from build123d import *

# Parameters (mm, degrees)
F0_W     = 7.8232
F0_H     = 6.35
F0_W_2   = 69.85
F0_H_2   = 3.175
F0_W_3   = 55.9308
F0_H_3   = 69.85
F0_W_4   = 7.7978
F0_H_4   = 12.7
F0_W_5   = 85.725
F1_DEPTH = 25.4
F0_W_6   = 2.8702
F0_H_5   = 5.1918955931
F0_W_7   = 66.0908
F0_H_6   = 4.9097025247
F0_H_7   = 13.4315382606
F0_W_8   = 16.764
F0_H_8   = 0.762
F2_DEPTH = 6.35


with BuildPart() as f1:
    # F0 (on Front) → F1 (new body)
    with BuildSketch(Plane.XZ):
        with Locations((148.4884, 43.5362195122)):
            Rectangle(F0_W, F0_H)
        with Locations((109.6518, 43.5362195122)):
            Rectangle(F0_W_2, F0_H)
        with Locations((148.4884, 38.7737195122)):
            Rectangle(F0_W, F0_H_2)
        with Locations((46.7614, 43.5362195122)):
            Rectangle(F0_W_3, F0_H)
        with Locations((109.6518, 38.7737195122)):
            Rectangle(F0_W_2, F0_H_2)
        with Locations((148.4884, 2.2612195122)):
            Rectangle(F0_W, F0_H_3)
        with Locations((46.7614, 38.7737195122)):
            Rectangle(F0_W_3, F0_H_2)
        with Locations((148.4884, -34.2512804878)):
            Rectangle(F0_W, F0_H_2)
        with Locations((-70.8279, 43.5362195122)):
            Rectangle(F0_W_4, F0_H)
        Polygon((74.7268, -2.1837804878), (74.7268, 37.1862195122), (18.796, 37.1862195122), (18.796, 3.0081151053), (18.796, -2.1837804878), align=None)
        with Locations((109.6518, -34.2512804878)):
            Rectangle(F0_W_2, F0_H_2)
        with Locations((148.4884, -39.0137804878)):
            Rectangle(F0_W, F0_H)
        with Locations((-109.6518, 43.5362195122)):
            Rectangle(F0_W_2, F0_H)
        with Locations((-70.8279, 38.7737195122)):
            Rectangle(F0_W_4, F0_H_2)
        with Locations((46.7614, -8.5337804878)):
            Rectangle(F0_W_3, F0_H_4)
        with Locations((109.6518, -39.0137804878)):
            Rectangle(F0_W_2, F0_H)
        Polygon((18.796, -32.6637804878), (74.7268, -32.6637804878), (74.7268, -14.8837804878), (18.796, -14.8837804878), (18.796, -28.3153187484), align=None)
        with Locations((46.7614, -34.2512804878)):
            Rectangle(F0_W_3, F0_H_2)
        with Locations((-148.4884, 43.5362195122)):
            Rectangle(F0_W, F0_H)
        with Locations((-109.6518, 38.7737195122)):
            Rectangle(F0_W_2, F0_H_2)
        Polygon((-66.929, 2.7259220369), (-66.929, 37.1862195122), (-74.7268, 37.1862195122), (-74.7268, -2.1837804878), (-66.929, -2.1837804878), align=None)
        with Locations((46.7614, -39.0137804878)):
            Rectangle(F0_W_3, F0_H)
        with Locations((-148.4884, 38.7737195122)):
            Rectangle(F0_W, F0_H_2)
        with Locations((-24.0665, -39.0137804878)):
            Rectangle(F0_W_5, F0_H)
        Polygon((-74.7268, -32.6637804878), (-66.929, -32.6637804878), (-66.929, -28.3153187484), (-66.929, -14.8837804878), (-74.7268, -14.8837804878), align=None)
        with Locations((-70.8279, -34.2512804878)):
            Rectangle(F0_W_4, F0_H_2)
        with Locations((-148.4884, 2.2612195122)):
            Rectangle(F0_W, F0_H_3)
        with Locations((-70.8279, -8.5337804878)):
            Rectangle(F0_W_4, F0_H_4)
        with Locations((-70.8279, -39.0137804878)):
            Rectangle(F0_W_4, F0_H)
        with Locations((-109.6518, -34.2512804878)):
            Rectangle(F0_W_2, F0_H_2)
        with Locations((-148.4884, -34.2512804878)):
            Rectangle(F0_W, F0_H_2)
        with Locations((-109.6518, -39.0137804878)):
            Rectangle(F0_W_2, F0_H)
        with Locations((-148.4884, -39.0137804878)):
            Rectangle(F0_W, F0_H)
    extrude(amount=F1_DEPTH)

    # F0 (on Front) → F2 (join)
    with BuildSketch(Plane.XZ):
        with Locations((-24.0665, 43.5362195122)):
            Rectangle(F0_W_5, F0_H)
        with Locations((-70.8279, 43.5362195122)):
            Rectangle(F0_W_4, F0_H)
        with Locations((-24.0665, 38.7737195122)):
            Rectangle(F0_W_5, F0_H_2)
        with Locations((-70.8279, 38.7737195122)):
            Rectangle(F0_W_4, F0_H_2)
        Polygon((18.796, 3.0081151053), (18.796, 37.1862195122), (-66.929, 37.1862195122), (-66.929, 2.7259220369), (-0.8382, 2.7259220369), (-0.8382, 3.0081151053), (15.9258, 3.0081151053), align=None)
        with Locations((17.3609, 0.4121673088)):
            Rectangle(F0_W_6, F0_H_5)
        Polygon((18.796, -14.8837804878), (18.796, -2.1837804878), (15.9258, -2.1837804878), (15.9258, -2.9457804878), (15.9258, -14.8837804878), align=None)
        Polygon((-66.929, -32.6637804878), (18.796, -32.6637804878), (18.796, -28.3153187484), (15.9258, -28.3153187484), (-0.8382, -28.3153187484), (-66.929, -28.3153187484), align=None)
        with Locations((-24.0665, -34.2512804878)):
            Rectangle(F0_W_5, F0_H_2)
        with Locations((-33.8836, 0.2710707746)):
            Rectangle(F0_W_7, F0_H_6)
        Polygon((15.9258, -2.1837804878), (15.9258, 3.0081151053), (-0.8382, 3.0081151053), (-0.8382, 2.7259220369), (-0.8382, -2.1837804878), align=None)
        with Locations((17.3609, -21.5995496181)):
            Rectangle(F0_W_6, F0_H_7)
        with Locations((7.5438, -2.5647804878)):
            Rectangle(F0_W_8, F0_H_8)
        Polygon((-0.8382, -2.1837804878), (-66.929, -2.1837804878), (-66.929, -14.8837804878), (-0.8382, -14.8837804878), (-0.8382, -2.9457804878), align=None)
        with Locations((7.5438, -21.5995496181)):
            Rectangle(F0_W_8, F0_H_7)
        with Locations((-33.8836, -21.5995496181)):
            Rectangle(F0_W_7, F0_H_7)
    extrude(amount=F2_DEPTH)


solid = f1.part
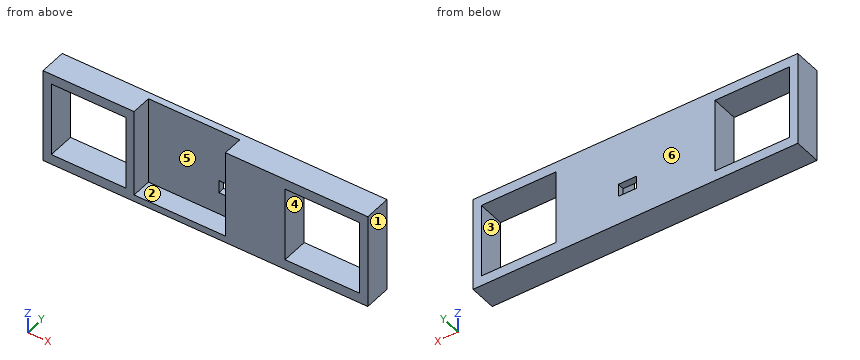
The model under review builds one solid part; all positions refer to its coordinate system, in mm. Face numbers are marked on the shaded views. A direction names the side the tool comes from. Round coordinates to 2 decimals unless told otherwise and drop trailing zeros. Write each loop counter-clockwise with the first axis right and the second up, starting at its lowest first coordinate (ties: lowest second). Pieces come first, ordered by that corner, then holes. Notation, with made-up numbers: M 54,55 L 113,55 A27 ccw 113,77 Z; hole C 54.25,-9 d1. An arc over 180 degrees is marked long. Answer as CSV lines item,"result". Start each with the question number.
Q1. The part is to be moulded in two halves that separate along Z. For the marked faces 1, 2 and 3, say which applies: +Z half, -Z half, draft (parallel to the pull), parting line (faces both ways), or undercut.
Q2. Consider section C-C, the plane y = -3.25. Give the boundary of the cut face in (x, z).
Q3. Consider section B-B, the plane x = -78. Give the boundary of the cut face in (y, z), then the cut area to 3 significant figures.
Q4. Clearance check with flat-ended pins moving along their axes: P1, Ø5.5, axis at x = -33.5, y = -16.5, coming from the +Z side; P2, Ø3, axis at x = -22.5, z = 10.5, coming from the -Y side. State where each tip first meets the part, or that it passes through.
Q5. Tool access review of the marked faces 4, 5 and 6: name each direction out of +Z, -Z, +X, -X, +Y, -Y from which nothing blocks a thin tool from reaching the whole face with its end or side.
Q6. Consider section D-D, the plane y = -22.25. Give the boundary of the cut face in (x, z).
Q7. Consider section A-A, the plane z = 11. Give the boundary of the cut face in (x, y), then the cut area to 3 significant figures.
Q8. Wall thickness on line 1 along X through (y, z) = (-13.5, 26.5); line 2 along X through (y, z) = (-0.75, 29); line 3 along X through (y, z) = (-4, -9): over which ranges is each line inside the solid? List them lowest first.
Result set:
1,face 1,"draft"
1,face 2,"+Z half"
1,face 3,"undercut"
2,outline,"M -152.4,-42.19 L 152.4,-42.19 L 152.4,46.71 L -152.4,46.71 Z; hole M -144.58,-32.66 L -74.73,-32.66 L -74.73,37.19 L -144.58,37.19 Z; hole M -0.84,-14.88 L 15.93,-14.88 L 15.93,-2.95 L -0.84,-2.95 Z; hole M 74.73,-32.66 L 144.58,-32.66 L 144.58,37.19 L 74.73,37.19 Z"
3,outline,"M -25.4,-42.19 L 0,-42.19 L 0,-32.66 L -25.4,-32.66 Z; M -25.4,37.19 L 0,37.19 L 0,46.71 L -25.4,46.71 Z"
3,area,"484 mm²"
4,P1,"stops at z = -35.84"
4,P2,"stops at y = -6.35"
5,face 4,"+Y, -Y"
5,face 5,"+Z, -Y"
5,face 6,"+Z, -Z, +X, -X, +Y"
6,outline,"M -152.4,-42.19 L 152.4,-42.19 L 152.4,46.71 L 18.8,46.71 L 18.8,-35.84 L -66.93,-35.84 L -66.93,46.71 L -152.4,46.71 Z; hole M -144.58,-32.66 L -74.73,-32.66 L -74.73,37.19 L -144.58,37.19 Z; hole M 74.73,-32.66 L 144.58,-32.66 L 144.58,37.19 L 74.73,37.19 Z"
7,outline,"M -152.4,-25.4 L -144.58,-25.4 L -144.58,0 L -152.4,0 Z; M -74.73,-25.4 L -66.93,-25.4 L -66.93,-6.35 L 18.8,-6.35 L 18.8,-25.4 L 74.73,-25.4 L 74.73,0 L -74.73,0 Z; M 144.58,-25.4 L 152.4,-25.4 L 152.4,0 L 144.58,0 Z"
7,area,"2,560 mm²"
8,line 1,"x = -152.4 to -144.58, -74.73 to -66.93, 18.8 to 74.73, 144.58 to 152.4"
8,line 2,"x = -152.4 to -144.58, -74.73 to 74.73, 144.58 to 152.4"
8,line 3,"x = -152.4 to -144.58, -74.73 to -0.84, 15.93 to 74.73, 144.58 to 152.4"
